from build123d import *

# Parameters (mm, degrees)
EXTRUDE_THIN1_DEPTH = 50
FILLET1_R           = 10
CUT_EXTRUDE1_DEPTH  = 10
SKETCH3_R           = 7
CUT_EXTRUDE2_DEPTH  = 10


with BuildPart() as part:
    # Sketch1 → Extrude-Thin1 (new body)
    with BuildSketch(Plane(origin=(0, 0, 0), x_dir=(0, 0, -1), z_dir=(1, 0, 0))):
        Polygon((0, 0), (100, 0), (100, 100), (110, 100), (110, -10), (0, -10), align=None)
    extrude(amount=EXTRUDE_THIN1_DEPTH)

    # Fillet1
    fillet1_edges = [part.edges().sort_by_distance(p)[0] for p in [
        (50, -5, 0),
        (0, -5, 0),
        (0, 100, -105),
        (50, 100, -105),
    ]]
    fillet(fillet1_edges, radius=FILLET1_R)

    # Sketch2 → Cut-Extrude1 (cut)
    with BuildSketch(Plane.XY.offset(-100)):
        with BuildLine():
            Line((30.184472994, 77.392944228), (30.184472994, 42.136183713))
            ThreePointArc((30.184472994, 42.136183713), (25, 36.951710719), (19.815527006, 42.136183713))
            Line((19.815527006, 42.136183713), (19.815527006, 77.392944228))
            ThreePointArc((19.815527006, 77.392944228), (25, 82.577417222), (30.184472994, 77.392944228))
        make_face()
    extrude(amount=-CUT_EXTRUDE1_DEPTH, mode=Mode.SUBTRACT)

    # Sketch3 → Cut-Extrude2 (cut)
    with BuildSketch(Plane(origin=(0, 0, 0), x_dir=(1, 0, 0), z_dir=(0, 1, 0))):
        with Locations(Location((25, 25.15267025, 0), (0, 0, 270))):
            Circle(SKETCH3_R)
        with Locations(Location((25, 61.300395832, 0), (0, 0, 270))):
            Circle(SKETCH3_R)
    extrude(amount=-CUT_EXTRUDE2_DEPTH, mode=Mode.SUBTRACT)


solid = part.part
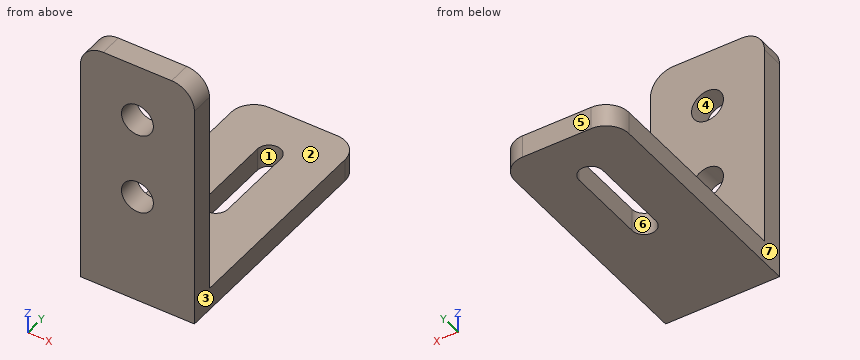
Input: part model. Units: mm. Frame: model coordinates. Face numbers are marked on the shaded views. A direction names the side the tool comes from. Give positions to 0.01 mm unless a question says otherwise; leave off trailing zeros. Order: outer loops, then holes, each group sorted by start corner. A loop starts at its lowest first (then second) coordinate and runs counter-clockwise, first axis right, second up. Notation, with made-up numbers: (-7.75, 16) - (42.25, 16) arc R19 ccw to (42.25, 38) - close; hole circle Ø2 at (36, 87). An arc over 180 degrees is marked (long way). Answer as a JSON object with one key per item and string values. Group by question number.
Q1. Cut plane A-A, the plane y = 64. Output: boundary loops of the cut face in (x, z).
Q2. Mould query, pull axis X, two halves, no side actions, for the marked faces 4, 5, 6 and 7. Classes: pulls with the +X half, pulls with the -X half, needs draft (parallel to the pull), parting line crosses it, or undercut.
Q3. First-contact query: pin 1 Ø3 at (x, y) = (19.5, 75) entering from +Z; pin 2 Ø8 at (x, z) = (27, -78) entering from +Y; pin 3 Ø2 at (x, y) = (28.5, 61) entering from -Z. Flat tips, straight axial feed; report the tip coordinate or a pass-through.
Q4. Set-up query: the marked faces 1, 2 and 3. Return all of +Z, -Z, +X, -X, +Y, -Y with unobstructed straight access to the full face (end or side cutting, diameter ignored); none if empty.
Q5. Cut plane C-C, the plane z = -57. Output: boundary loops of the cut face in (x, y), then the cut area to 3 significant figures.
Q6. Cut plane B-B, the plane x = 25. Output: boundary loops of the cut face in (y, z), then the cut area to 3 significant figures.
Q7. Cut plane D-D, the plane x = 44. Output: boundary loops of the cut face in (y, z).
Q8. Line query: probe 1 along Y at (x, z) = (25.5, -90.5); probe 2 along Z at (x, y) = (30.5, 33). Output: solid intervals per line, ascending.
Results:
{
 "1": {"outline": "(0, -110) - (19.82, -110) - (19.82, -100) - (0, -100) - close; (30.18, -110) - (50, -110) - (50, -100) - (30.18, -100) - close"},
 "2": {"face 4": "undercut", "face 5": "needs draft", "face 6": "undercut", "face 7": "pulls with the -X half"},
 "3": {"pin 1": "z = -100", "pin 2": "y = 0", "pin 3": "through"},
 "4": {"face 1": "+Z, -Z", "face 2": "+Z, +X, -X, +Y", "face 3": "+Z, -Z, +X, +Y, -Y"},
 "5": {"outline": "(0, -10) - (19.48, -10) - (19.48, 0) - (0, 0) - close; (30.52, -10) - (50, -10) - (50, 0) - (30.52, 0) - close", "area": "390 mm^2"},
 "6": {"outline": "(-10, -110) - (36.95, -110) - (36.95, -100) - (0, -100) - (0, -68.3) - (-10, -68.3) - close; (-10, -54.3) - (0, -54.3) - (0, -32.15) - (-10, -32.15) - close; (-10, -18.15) - (0, -18.15) - (0, 0) - (-10, 0) - close; (82.58, -110) - (100, -110) - (100, -100) - (82.58, -100) - close", "area": "1,360 mm^2"},
 "7": {"outline": "(-10, -110) - (99.17, -110) - (99.17, -100) - (0, -100) - (0, -0.83) - (-10, -0.83) - close"},
 "8": {"probe 1": "-10 to 0", "probe 2": "-110 to -100"}
}
